Autodesk Inventor part; units mm, degrees
ref_plane "YZ Plane" through (0, 0, 0) normal (1, 0, 0) x (0, 1, 0)
ref_plane "XZ Plane" through (0, 0, 0) normal (0, 1, 0) x (-1, 0, 0)
ref_plane "XY Plane" through (0, 0, 0) normal (0, 0, 1) x (1, 0, 0)
sketch "Sketch1" plane through (0, 0, 0) normal (0, 0, 1) x (1, 0, 0)
  line L0 (3, 1) -> (3, 0)
  line L1 (3, 0) -> (-3, 0)
  line L2 (-3, 0) -> (-3, 1)
  line L3 (3, 1) -> (-3, 1)
  point P0 (0, 0)
  point P1 (0, 0)
  dimension "d0" = 6
  dimension "d6" = 1
extrude "Extrusion1" add sketch "Sketch1" along normal mid plane 17
sketch "Sketch2" plane through (-3, 0, 8.5) normal (0, -1, 0) x (1, 0, 0)
  line L0 (0, -5.5) -> (5, -5.5)
  line L1 (5, -5.5) -> (5, -4.5)
  line L2 (1, -4.5) -> (0, -4.5)
  line L3 (0, -4.5) -> (0, -5.5)
  line L4 (6, -3.5) -> (1, -3.5)
  line L5 (1, -3.5) -> (1, -4.5)
  line L6 (5, -4.5) -> (6, -4.5)
  line L7 (6, -4.5) -> (6, -3.5)
  line L8 (0, -17) -> (0, 0)
  line L9 (6, 0) -> (6, -17)
  line L10 (6, 0) -> (0, 0)
  line L11 (6, 0) -> (0, 0)
  line L12 (0, -17) -> (0, 0)
  line L13 (0, -17) -> (6, -17)
  line L14 (6, 0) -> (6, -17)
  line L15 (-1.2, -8.5) -> (7.2, -8.5)
  line L16 (5, -11.5) -> (5, -12.5)
  line L17 (1, -12.5) -> (0, -12.5)
  line L18 (0, -12.5) -> (0, -11.5)
  line L19 (6, -13.5) -> (1, -13.5)
  line L20 (1, -13.5) -> (1, -12.5)
  line L21 (5, -12.5) -> (6, -12.5)
  line L22 (6, -12.5) -> (6, -13.5)
  line L23 (0, -11.5) -> (5, -11.5)
  point P0 (3, -8.5)
  dimension "d7" = 1
  dimension "d8" = 1
  dimension "d9" = 2
  dimension "d10" = 3.5
extrude "Extrusion2" add sketch "Sketch2" along normal blind 2 contours L3 L2 L5 L4 L7 L6 L1 L0 | L23 L16 L21 L9 L19 L20 L17 L8
sketch "Sketch3" plane through (-3, 0, 3) normal (0, -1, 0) x (1, 0, 0)
  line L0 (6, 1) -> (5, 1)
  line L1 (5, 1) -> (5, 0)
  line L2 (5, 0) -> (0, 0)
  line L3 (0, -6) -> (0, 0)
  line L4 (0, -6) -> (5, -6)
  line L5 (5, -6) -> (5, -7)
  line L6 (5, -7) -> (6, -7)
  line L7 (6, 1) -> (6, -7)
  line L8 (4, -1.5) -> (0, -1.5)
  line L9 (0, -1.5) -> (0, -4.5)
  line L10 (0, -4.5) -> (4, -4.5)
  line L11 (4, -4.5) -> (4, -1.5)
  line L12 (0, -6) -> (0, 0)
  line L13 (-1.2, -3) -> (7.2, -3)
  point P0 (3, -3)
  point P1 (0, -3)
  dimension "d13" = 4
  dimension "d14" = 3
extrude "Extrusion3" cut sketch "Sketch3" against normal through all contours L13 L3 L8 L11 | L11 L10 L3 L13
sketch "Sketch4" plane through (-3, 1, 8.5) normal (0, 1, 0) x (1, 0, 0)
  line L0 (6, 2) -> (4, 2)
  line L1 (4, 2) -> (4, 15)
  line L2 (4, 15) -> (6, 15)
  line L3 (6, 15) -> (6, 2)
  line L4 (-1.2, 8.5) -> (7.2, 8.5)
  line L5 (6, 17) -> (6, 0)
  line L6 (4, 10) -> (4, 7)
  point P0 (3, 8.5)
  dimension "d17" = 13
extrude "Extrusion4" add sketch "Sketch4" along normal blind 2
properties part number "track" material "Rubber"
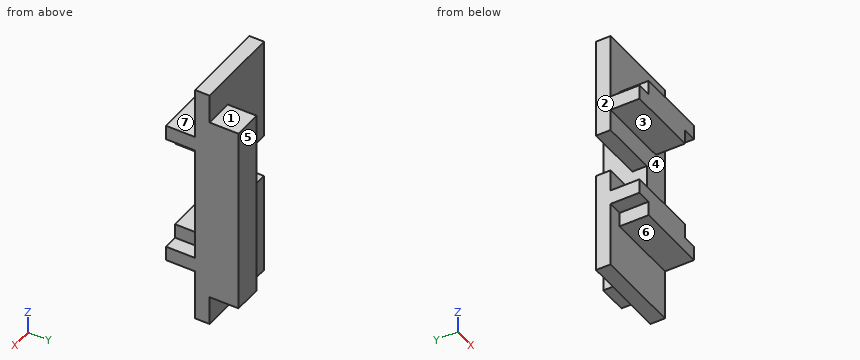
Part model, mm, in its own coordinate system. Face numbers are marked on the shaded views. A direction names the side the tool comes from. Coordinates: 2 decimals unless noted, no trailing zeros. Order: outer loops, then holes, each group sorted by start corner. A loop starts at its lowest first (then second) coordinate and runs counter-clockwise, first axis right, second up. Notation, with made-up numbers: (-13.75, 14.5) -> (-3.75, 14.5) arc R15 ccw to (-3.75, 30.5) -> close; hole circle Ø2 at (74.5, -20.5). An arc over 180 degrees is marked (long way). Put each result on its own line as item: value. Start each with the question number.
(1) Probe line 1 along Z through (x, y) = (2.75, -0.85); line 2 along Z through (x, y) = (-1.5, 0.3); line 3 along X through (y, z) = (1.6, -1.75). List the from-to ranges inside material, lowest first. Write a range as [from, to].
(2) Pin check, flat tips, straight feed: pin 1 Ø1.5 at (y, z) = (2, -1.5) entering from -X; pin 2 Ø0.8 at (y, z) = (-1, -3.5) entering from +X; pin 3 Ø1.8 at (x, z) = (-1.5, -6) entering from +Y. Stop position of each tip, or through.
(3) Band-saw the part on D-D (x = 2.3). Give the cut face in (y, z).
(4) Band-saw the part on B-B (z = 3.75). Give the cut face in (x, y).
(5) Mould opens along Z. For the marked faces 4, 5, 6 and 7 say: pulls with the +Z half, pulls with the -Z half, needs draft (parallel to the pull), parting line crosses it, or undercut.
(6) Band-saw the part on C-C (y = 0.2). Give the cut face in (x, z), then the cut area to 3 significant figures.
(7) Which spindle directions (+Z, -Z, +X, -X, +Y, -Y) get a long thin tool onto all of the face, cutting with end or side? Do the marked faces 1, 2 and 3. Say none if no direction does.
(8) Band-saw the part on A-A (y = -0.65). Give the cut face in (x, z).
Determined:
1. line 1: z = [-5, -4], [4, 5]
1. line 2: z = [-8.5, -1.5], [1.5, 8.5]
1. line 3: x = [1, 3]
2. pin 1: stops at x = 1
2. pin 2: stops at x = 2
2. pin 3: stops at y = 1
3. outline: (-2, -5) -> (0, -5) -> (0, -8.5) -> (1, -8.5) -> (1, -6.5) -> (3, -6.5) -> (3, 6.5) -> (1, 6.5) -> (1, 8.5) -> (0, 8.5) -> (0, 5) -> (-2, 5) -> (-2, 4) -> (0, 4) -> (0, -4) -> (-2, -4) -> close
4. outline: (-3, -2) -> (2, -2) -> (2, 0) -> (3, 0) -> (3, 3) -> (1, 3) -> (1, 1) -> (-3, 1) -> close
5. face 4: undercut
5. face 5: needs draft
5. face 6: pulls with the -Z half
5. face 7: pulls with the +Z half
6. outline: (-3, -8.5) -> (3, -8.5) -> (3, 8.5) -> (-3, 8.5) -> (-3, 1.5) -> (1, 1.5) -> (1, -1.5) -> (-3, -1.5) -> close
6. area: 90.0 mm²
7. face 1: +Z, +X, -X, +Y
7. face 2: +Z, -Z, -X, +Y, -Y
7. face 3: +X, -X, -Y
8. outline: (-3, -4) -> (-2, -4) -> (-2, -5) -> (3, -5) -> (3, -4) -> (2, -4) -> (2, -3) -> (-3, -3) -> close; (-3, 3) -> (2, 3) -> (2, 4) -> (3, 4) -> (3, 5) -> (-2, 5) -> (-2, 4) -> (-3, 4) -> close
